from build123d import *

# Parameters (mm, degrees)
SKETCH_1_W          = 37
SKETCH_1_H          = 21
EXTRUDE_1_DEPTH     = 3
SKETCH_2_W          = 6
SKETCH_2_H          = 2
CUT_EXTRUDE_1_DEPTH = 10
SKETCH_2_10_W       = 6
SKETCH_2_10_H       = 2
CUT_EXTRUDE_2_DEPTH = 2.5
SKETCH_5_W          = 21
SKETCH_5_H          = 1
EXTRUDE_2_DEPTH     = 1
SKETCH_7_W          = 37
SKETCH_7_H          = 1
EXTRUDE_3_DEPTH     = 1
SKETCH_8_W          = 21
SKETCH_8_H          = 1
EXTRUDE_4_DEPTH     = 1


with BuildPart() as part:
    # Эскиз1 → Бобышка-Вытянуть1 (new body)
    with BuildSketch(Plane(origin=(0, 0, 0), x_dir=(1, 0, 0), z_dir=(0, 1, 0))):
        with Locations((18.5, -10.5)):
            Rectangle(SKETCH_1_W, SKETCH_1_H)
    extrude(amount=EXTRUDE_1_DEPTH)

    # Эскиз2 → Вырез-Вытянуть1 (cut)
    with BuildSketch(Plane.XZ):
        with Locations((6.5, 12.5)):
            Rectangle(SKETCH_2_W, SKETCH_2_H)
        with Locations((6.5, 8.5)):
            Rectangle(SKETCH_2_W, SKETCH_2_H)
        with Locations((14.5, 12.5)):
            Rectangle(SKETCH_2_W, SKETCH_2_H)
        with Locations((14.5, 8.5)):
            Rectangle(SKETCH_2_W, SKETCH_2_H)
        with Locations((22.5, 12.5)):
            Rectangle(SKETCH_2_W, SKETCH_2_H)
        with Locations((22.5, 8.5)):
            Rectangle(SKETCH_2_W, SKETCH_2_H)
        with Locations((30.5, 12.5)):
            Rectangle(SKETCH_2_W, SKETCH_2_H)
        with Locations((30.5, 8.5)):
            Rectangle(SKETCH_2_W, SKETCH_2_H)
    extrude(amount=-CUT_EXTRUDE_1_DEPTH, mode=Mode.SUBTRACT)

    # Эскиз2<10> → Вырез-Вытянуть2 (cut)
    with BuildSketch(Plane.XZ):
        with Locations((6.5, 10.5)):
            Rectangle(SKETCH_2_10_W, SKETCH_2_10_H)
        with Locations((14.5, 10.5)):
            Rectangle(SKETCH_2_10_W, SKETCH_2_10_H)
        with Locations((22.5, 10.5)):
            Rectangle(SKETCH_2_10_W, SKETCH_2_10_H)
        with Locations((30.5, 10.5)):
            Rectangle(SKETCH_2_10_W, SKETCH_2_10_H)
    extrude(amount=-CUT_EXTRUDE_2_DEPTH, mode=Mode.SUBTRACT)

    # Эскиз5 → Бобышка-Вытянуть2 (add)
    with BuildSketch(Plane(origin=(37, 0, 0), x_dir=(0, 0, -1), z_dir=(1, 0, 0))):
        with Locations((-10.5, 1.5)):
            Rectangle(SKETCH_5_W, SKETCH_5_H)
    extrude(amount=EXTRUDE_2_DEPTH)

    # Эскиз7 → Бобышка-Вытянуть3 (add)
    with BuildSketch(Plane(origin=(0, 0, 0), x_dir=(-1, 0, 0), z_dir=(0, 0, -1))):
        with Locations((-18.5, 1.5)):
            Rectangle(SKETCH_7_W, SKETCH_7_H)
    extrude(amount=EXTRUDE_3_DEPTH)

    # Эскиз8 → Бобышка-Вытянуть4 (add)
    with BuildSketch(Plane.ZY):
        with Locations((10.5, 1.5)):
            Rectangle(SKETCH_8_W, SKETCH_8_H)
    extrude(amount=EXTRUDE_4_DEPTH)


solid = part.part
Work out the finished part from the listing and answer in its coordinate system (mm). A direction names the side the tool comes from. Round coordinates to 2 decimals unless told otherwise and drop trailing zeros. Write each loop counter-clockwise with the first axis right and the second up, starting at its lowest first coordinate (ties: lowest second). Pieces come first, ordered by that corner, then holes.
1) Straight lines are drawn through the part: line 1 (X direction, y = 1.45, z = 8); line 2 (X direction, y = 0.4, z = 11.5); line 3 (Z direction, x = 24, y = 0.85). For each, find the intervals that lie inside material, in ascending order.
2) A cutting plane is placed at C-C (z = 10.5). Give the vertices of the cut face in (x, y), plus the area to 3 significant figures.
3) A cutting plane is placed at A-A (y = 1.6). Give the vertices of the cut face in (x, z).
4) A cutting plane is placed at B-B (x = 25). Give the vertices of the cut face in (y, z).
5) A tool of negligible diameter and unlimited length cuts with its end or side. For faces 1 (the flat face through (30, 2.5, 11)), 2 (the flat face through (18.2, 0.5, 0)), 3 (the flat face through (22, 1, 7.5)), 4 (the flat face through (18.2, 2.5, 0)), 5 (the flat face through (37.5, 1, 10.6)), from which of +Z, -Z, +X, -X, +Y, -Y can it reach the whole face along a straight path? Write none if from no direction.
6) A cutting plane is placed at D-D (z = 14.25). Give the vertices of the cut face in (x, y), plus the area to 3 significant figures.
7) Given pin 1 Ø1 at (x, z) = (30.5, 10) entering from -Y; pin 2 Ø0.8 at (y, z) = (1.5, -0.5) entering from -X; pin 3 Ø0.5 at (x, y) = (26, 2.5) entering from -Z, each flat-ended and moving along its own axis, determine where each tip first touches the part or whether it passes through.
Completed:
1. line 1: x = -1 to 3.5, 9.5 to 11.5, 17.5 to 19.5, 25.5 to 27.5, 33.5 to 38
1. line 2: x = 0 to 3.5, 9.5 to 11.5, 17.5 to 19.5, 25.5 to 27.5, 33.5 to 37
1. line 3: z = 0 to 7.5, 13.5 to 21
2. outline: (-1, 1) - (0, 1) - (0, 0) - (3.5, 0) - (3.5, 2.5) - (9.5, 2.5) - (9.5, 0) - (11.5, 0) - (11.5, 2.5) - (17.5, 2.5) - (17.5, 0) - (19.5, 0) - (19.5, 2.5) - (25.5, 2.5) - (25.5, 0) - (27.5, 0) - (27.5, 2.5) - (33.5, 2.5) - (33.5, 0) - (37, 0) - (37, 1) - (38, 1) - (38, 2) - (37, 2) - (37, 3) - (0, 3) - (0, 2) - (-1, 2) - close
2. area: 53.0 mm2
3. outline: (-1, 0) - (0, 0) - (0, -1) - (37, -1) - (37, 0) - (38, 0) - (38, 21) - (-1, 21) - close; hole (3.5, 7.5) - (9.5, 7.5) - (9.5, 13.5) - (3.5, 13.5) - close; hole (11.5, 7.5) - (17.5, 7.5) - (17.5, 13.5) - (11.5, 13.5) - close; hole (19.5, 7.5) - (25.5, 7.5) - (25.5, 13.5) - (19.5, 13.5) - close; hole (27.5, 7.5) - (33.5, 7.5) - (33.5, 13.5) - (27.5, 13.5) - close
4. outline: (0, 0) - (1, 0) - (1, -1) - (2, -1) - (2, 0) - (3, 0) - (3, 7.5) - (0, 7.5) - close; (0, 13.5) - (3, 13.5) - (3, 21) - (0, 21) - close; (2.5, 9.5) - (3, 9.5) - (3, 11.5) - (2.5, 11.5) - close
5. face 1: -Y
5. face 2: -Z, +X, -X, -Y
5. face 3: +Y, -Y
5. face 4: -Z, +X, -X, +Y
5. face 5: +Z, -Z, +X, -Y
6. outline: (-1, 1) - (0, 1) - (0, 0) - (37, 0) - (37, 1) - (38, 1) - (38, 2) - (37, 2) - (37, 3) - (0, 3) - (0, 2) - (-1, 2) - close
6. area: 113 mm2
7. pin 1: stops at y = 2.5
7. pin 2: stops at x = 0
7. pin 3: stops at z = 0
